Check sheet for the modelled part. Datum: model origin and axes. Units: mm. A direction names the side the tool comes from. Round coordinates to 2 decimals unless told otherwise and drop trailing zeros. Loops run counter-clockwise (first coordinate to the right, second up) from the corner with the lowest first, then second, coordinate; pieces in that order, holes last. Notation, with made-up numbers: (8, 48) - (50, 48) arc R19 cw to (50, 72) - close; hole circle Ø3 at (-35.5, 68.5). An arc over 180 degrees is marked (long way). Answer in a Markdown table with one row per item. Add a question column.
(1) Cross-section at B-B on y = -22.5. Enter the section's corners in (x, z), then the cut area to 3 significant figures.
(2) Cross-section at A-A on x = -60. Enter the section's corners in (y, z).
(3) Cross-section at D-D on x = -30.5. Enter the section's corners in (y, z), then the cut area to 3 significant figures.
(4) Access from +Z, -Z, +X, -X, +Y, -Y to the whole of each face (thin tool, end or side, straight path). Record for faces 1 (the flat face through (1, 0, 58)), 2 (the flat face through (35, -25, 58)), 3 (the flat face through (75, -3, 58)), 4 (the flat face through (-75, -3, 58)), 5 (the flat face through (65, -15, 58)).
(5) Cross-section at C-C on z = 98.5. Enter the section's corners in (x, y), then the cut area to 3 significant figures.
(6) Gauge pin test, flat ends, axial feed: pin 1 (9 mm diameter, centred on x = 60, y = 35.51, fed in from -Z); pin 2 (1 mm diameter, centred on x = 12, z = 93.5, fed in from +Y); pin 3 (6.5 mm diameter, centred on x = -60, y = 35.51, fed in from -Z). Record the tip position at first contact, or that the pin passes through.
(7) Thickness scan on line 1 along Y through (x, z) = (-60, 3); line 2 along Y through (x, z) = (57.5, 11); line 3 along Z through (x, y) = (-36, 5). Record the ranges inside material, lowest first.
(8) Mould release check, pull along Y, two halves, no side actions. Record for faces 6 (the flat face through (-35, -25, 58)), 7 (the flat face through (-1, -10, 58)), 8 (the flat face through (1, 70, 112)): +Y half, -Y half, draft (parallel to the pull), parting line (faces both ways), or undercut.
from build123d import *

# Parameters (mm, degrees)
F1_DEPTH = 117
F2_W     = 150
F2_H     = 10
F3_DEPTH = 70
F4_R     = 4
F5_DEPTH = 139.1


with BuildPart() as f1:
    # F0 (on Top) → F1 (new body)
    with BuildSketch(Plane.XY):
        Polygon((-75, -30), (-35, -30), (-35, -20), (-65, -20), (-65, -10), (65, -10), (65, -20), (35, -20), (35, -30), (75, -30), (75, 0), (-75, 0), align=None)
    extrude(amount=F1_DEPTH)

    # F2 (on face) → F3 (join)
    with BuildSketch(Plane(origin=(0, 0, 0), x_dir=(-1, 0, 0), z_dir=(0, 1, 0))):
        with Locations((0, 112)):
            Rectangle(F2_W, F2_H)
        with Locations((0, 5)):
            Rectangle(F2_W, F2_H)
    extrude(amount=F3_DEPTH)

    # F4 (on face) → F5 (cut)
    with BuildSketch(Plane(origin=(0, 0, 0), x_dir=(1, 0, 0), z_dir=(0, 0, -1))):
        with Locations((-60, -35.509091)):
            Circle(F4_R)
        with Locations((60, -35.509091)):
            Circle(F4_R)
    extrude(amount=-F5_DEPTH, mode=Mode.SUBTRACT)


solid = f1.part
Answers:
| question | item | result |
|---|---|---|
| 1 | outline | (-75, 0) - (-35, 0) - (-35, 117) - (-75, 117) - close; (35, 0) - (75, 0) - (75, 117) - (35, 117) - close |
| 1 | area | 9,360 mm^2 |
| 2 | outline | (-30, 0) - (-20, 0) - (-20, 117) - (-30, 117) - close; (-10, 0) - (31.51, 0) - (31.51, 10) - (0, 10) - (0, 107) - (31.51, 107) - (31.51, 117) - (-10, 117) - close; (39.51, 0) - (70, 0) - (70, 10) - (39.51, 10) - close; (39.51, 107) - (70, 107) - (70, 117) - (39.51, 117) - close |
| 3 | outline | (-10, 0) - (70, 0) - (70, 10) - (0, 10) - (0, 107) - (70, 107) - (70, 117) - (-10, 117) - close |
| 3 | area | 2,570 mm^2 |
| 4 | face 1 | +X, -X, +Y |
| 4 | face 2 | +Z, -Z, -Y |
| 4 | face 3 | +Z, -Z, +X, +Y, -Y |
| 4 | face 4 | +Z, -Z, -X, +Y, -Y |
| 4 | face 5 | +Z, -Z |
| 5 | outline | (-75, -30) - (-35, -30) - (-35, -20) - (-65, -20) - (-65, -10) - (65, -10) - (65, -20) - (35, -20) - (35, -30) - (75, -30) - (75, 0) - (-75, 0) - close |
| 5 | area | 2,500 mm^2 |
| 6 | pin 1 | stops at z = 0 |
| 6 | pin 2 | stops at y = 0 |
| 6 | pin 3 | passes through |
| 7 | line 1 | y = -30 to -20, -10 to 31.51, 39.51 to 70 |
| 7 | line 2 | y = -30 to -20, -10 to 0 |
| 7 | line 3 | z = 0 to 10, 107 to 117 |
| 8 | face 6 | draft |
| 8 | face 7 | undercut |
| 8 | face 8 | +Y half |
